The drawing under review shows one solid part. Ordinate dimensions are in mm from its lowest x, y, z. A direction names the side the tool comes from. Give positions to 0.01 mm unless a question says otherwise; leave off trailing zeros. Write each loop counter-clockwise with the first axis right and the second up, starting at its lowest first coordinate (ties: lowest second). Pieces come first, ordered by that corner, then holes.
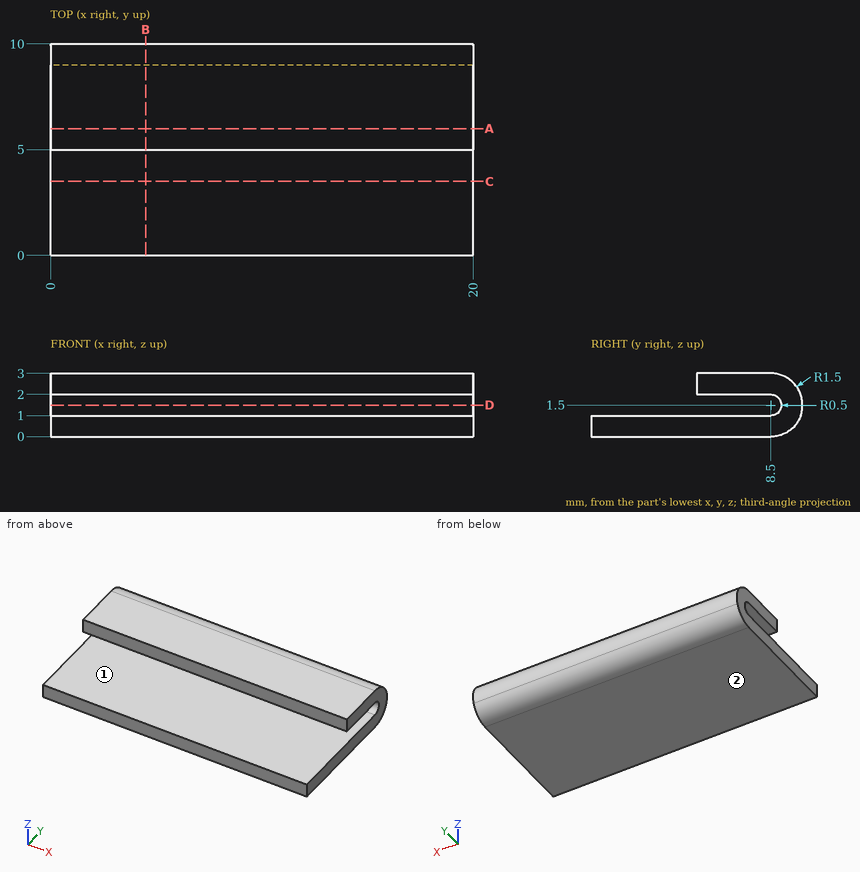
1) Consider section D-D, the plane z = 1.5. Give the boundary of the cut face in (x, y).
2) Consider section B-B, the plane x = 4.5. Give the boundary of the cut face in (y, z).
3) Consider section A-A, the plane y = 6. Give the boundary of the cut face in (x, z), then the cut area to 3 significant figures.
4) Consider section C-C, the plane y = 3.5. Give the boundary of the cut face in (x, z).
5) Insertion check: pin 1 (1.5 mm diameter, centred on y = 6.5, z = 2, fed in from -X); pin 2 (0.8 mm diameter, centred on x = 7.5, z = 2.5, fed in from -Y). Each pin has a flat end and moves straight along its axis. Give the tip position at first contact, or say it passes through.
6) To check wall thickness, follow probe 1 along Z at (x, y) = (14.75, 6.5); probe 2 along Z at (x, y) = (8.25, 0.75); probe 3 along Y at (x, z) = (4.5, 0.6). State the ranges of each line that lie inside material, in increasing order.
7) Tool access review of the marked faces 1 and 2: name each direction out of +Z, -Z, +X, -X, +Y, -Y from which nothing blocks a thin tool from reaching the whole face with its end or side.
Answer block:
1. outline: (0, 9) - (20, 9) - (20, 10) - (0, 10) - close
2. outline: (0, 0) - (8.5, 0) arc R1.5 ccw to (8.5, 3) - (5, 3) - (5, 2) - (8.5, 2) arc R0.5 cw to (8.5, 1) - (0, 1) - close
3. outline: (0, 0) - (20, 0) - (20, 1) - (0, 1) - close; (0, 2) - (20, 2) - (20, 3) - (0, 3) - close
3. area: 40.0 mm2
4. outline: (0, 0) - (20, 0) - (20, 1) - (0, 1) - close
5. pin 1: stops at x = 0
5. pin 2: stops at y = 5
6. probe 1: z = 0 to 1, 2 to 3
6. probe 2: z = 0 to 1
6. probe 3: y = 0 to 9.7
7. face 1: +X, -X, -Y
7. face 2: -Z, +X, -X, +Y, -Y
